Work out the finished part from the listing and answer in its coordinate system (mm). A direction names the side the tool comes from. Give positions to 0.01 mm unless a question says otherwise; leave off trailing zeros. Write each loop counter-clockwise with the first axis right and the second up, starting at its lowest first coordinate (ties: lowest second). Pieces come first, ordered by that corner, then holes. Notation, with made-up numbers: (75, 33) - (130, 33) arc R22 ccw to (130, 57) - close; hole circle Ø5 at (-6.5, 38.5). An arc over 180 degrees is marked (long way). Write item = value, one per line.
from build123d import *

# Parameters (mm, degrees)
BASE_FLANGE1_DEPTH                           = 19.5
SKETCH13_R                                   = 4
CUT_EXTRUDE6_DEPTH                           = 84.228219974
CUT_EXTRUDE7_DEPTH                           = 84.228219974
CUT_EXTRUDE7_DEPTH_BACK                      = 84.228219974
SKETCH33_R                                   = 8
CUT_EXTRUDE10_DEPTH                          = 10
SKETCH34_R                                   = 1.5
CUT_EXTRUDE11_DEPTH                          = 10
BOSS_EXTRUDE1_DEPTH                          = 3
TAB1_START                                   = -3
TAB1_DEPTH                                   = 3
CSK_FOR_M4_COUNTERSUNK_FLAT_HEAD_SCR_2_COUNT = 2
CSK_FOR_M4_COUNTERSUNK_FLAT_HEAD_SCR_2_PITCH = 39.597979746
CSK_FOR_M4_COUNTERSUNK_FLAT_HEAD_SCR_3_COUNT = 2
CSK_FOR_M4_COUNTERSUNK_FLAT_HEAD_SCR_3_PITCH = 56
CSK_FOR_M4_COUNTERSUNK_FLAT_HEAD_SCR_4_COUNT = 2
CSK_FOR_M4_COUNTERSUNK_FLAT_HEAD_SCR_4_PITCH = 39.597979746


# Read off the part's stored shape, not the designer's step: Tab1
# Sheet-metal steps are written as plain solids
with BuildPart() as part:
    # Sketch1 → Base-Flange1 (new, symmetric)
    with BuildSketch(Plane.XY):
        with BuildLine():
            Line((-28.21, 74.65), (-28.21, 2))
            ThreePointArc((-28.21, 2), (-27.624213562, 0.585786438), (-26.21, 0))
            Line((-26.21, 0), (26.21, 0))
            ThreePointArc((26.21, 0), (27.624213562, 0.585786438), (28.21, 2))
            Line((28.21, 2), (28.21, 74.65))
            Line((28.21, 74.65), (31.21, 74.65))
            Line((31.21, 74.65), (31.21, 2))
            ThreePointArc((31.21, 2), (29.745533906, -1.535533906), (26.21, -3))
            Line((26.21, -3), (-26.21, -3))
            ThreePointArc((-26.21, -3), (-29.745533906, -1.535533906), (-31.21, 2))
            Line((-31.21, 2), (-31.21, 74.65))
            Line((-31.21, 74.65), (-28.21, 74.65))
        make_face()
    extrude(amount=BASE_FLANGE1_DEPTH, both=True)

    # Sketch13 → Cut-Extrude6 (cut, through all)
    with BuildSketch(Plane(origin=(0, 0, 0), x_dir=(0, 0, -1), z_dir=(1, 0, 0))):
        with Locations((0, 32)):
            Circle(SKETCH13_R)
    extrude(amount=CUT_EXTRUDE6_DEPTH, mode=Mode.SUBTRACT)

    # Sketch15 → Cut-Extrude7 (cut, two sides: drawn at the far end of the back side and taken through both)
    with BuildSketch(Plane(origin=(0, 0, 0), x_dir=(0, 0, -1), z_dir=(1, 0, 0)).offset(-CUT_EXTRUDE7_DEPTH_BACK)):
        with BuildLine():
            Line((-19.5, 32), (-26.744382408, 32))
            Line((-26.744382408, 32), (-26.744382408, 87.632847334))
            Line((-26.744382408, 87.632847334), (26.744382408, 87.632847334))
            Line((26.744382408, 87.632847334), (26.744382408, 32))
            Line((26.744382408, 32), (19.5, 32))
            ThreePointArc((19.5, 32), (0, 51.5), (-19.5, 32))
        make_face()
        with BuildLine():
            Line((7.470480628, 19.147299148), (10, 14.795349466))
            ThreePointArc((10, 14.795349466), (10.176160856, 13.182152576), (9.097954318, 11.969342816))
            ThreePointArc((9.097954318, 11.969342816), (0, 10), (-9.097954318, 11.969342816))
            ThreePointArc((-9.097954318, 11.969342816), (-10.176160856, 13.182152576), (-10, 14.795349466))
            Line((-10, 14.795349466), (-7.470480628, 19.147299148))
            ThreePointArc((-7.470480628, 19.147299148), (-6.381394917, 20.037080634), (-4.975835097, 19.989959822))
            ThreePointArc((-4.975835097, 19.989959822), (0, 19), (4.975835097, 19.989959822))
            ThreePointArc((4.975835097, 19.989959822), (6.381394917, 20.037080634), (7.470480628, 19.147299148))
        make_face()
    extrude(amount=CUT_EXTRUDE7_DEPTH + CUT_EXTRUDE7_DEPTH_BACK, mode=Mode.SUBTRACT)

    # Sketch33 → Cut-Extrude10 (cut)
    with BuildSketch(Plane(origin=(-28.21, 0, 0), x_dir=(0, 0, -1), z_dir=(1, 0, 0))):
        with Locations((0, 32)):
            Circle(SKETCH33_R)
    extrude(amount=-CUT_EXTRUDE10_DEPTH, mode=Mode.SUBTRACT)

    # Sketch34 → Cut-Extrude11 (cut)
    with BuildSketch(Plane.ZY.offset(31.21)):
        with Locations((-11.490485194, 43.490485194)):
            Circle(SKETCH34_R)
        with Locations((11.490485194, 43.490485194)):
            Circle(SKETCH34_R)
        with Locations((11.490485194, 20.509514806)):
            Circle(SKETCH34_R)
        with Locations((-11.490485194, 20.509514806)):
            Circle(SKETCH34_R)
    extrude(amount=-CUT_EXTRUDE11_DEPTH, mode=Mode.SUBTRACT)

    # Sketch37 → Boss-Extrude1 (add)
    with BuildSketch(Plane.ZY.offset(31.21)):
        with BuildLine():
            Line((7.470480628, 19.147299148), (10, 14.795349466))
            ThreePointArc((10, 14.795349466), (10.176160856, 13.182152576), (9.097954318, 11.969342816))
            ThreePointArc((9.097954318, 11.969342816), (0, 10), (-9.097954318, 11.969342816))
            ThreePointArc((-9.097954318, 11.969342816), (-10.176160856, 13.182152576), (-10, 14.795349466))
            Line((-10, 14.795349466), (-7.470480628, 19.147299148))
            ThreePointArc((-7.470480628, 19.147299148), (-6.381394917, 20.037080634), (-4.975835097, 19.989959822))
            ThreePointArc((-4.975835097, 19.989959822), (0, 19), (4.975835097, 19.989959822))
            ThreePointArc((4.975835097, 19.989959822), (6.381394917, 20.037080634), (7.470480628, 19.147299148))
        make_face()
    extrude(amount=-BOSS_EXTRUDE1_DEPTH)

    # Tab1 outline → Tab1 (add)
    with BuildSketch(Plane.XZ.offset(3).offset(TAB1_START)):
        with BuildLine():
            Line((26.21, 19.5), (26.21, 23.195600876))
            ThreePointArc((26.21, 23.195600876), (0, 35), (-26.21, 23.195600876))
            Line((-26.21, 23.195600876), (-26.21, 19.5))
            Line((-26.21, 19.5), (26.21, 19.5))
        make_face()
        with BuildLine():
            Line((-26.21, -19.5), (-26.21, -23.195600876))
            ThreePointArc((-26.21, -23.195600876), (0, -35), (26.21, -23.195600876))
            Line((26.21, -23.195600876), (26.21, -19.5))
            Line((26.21, -19.5), (-26.21, -19.5))
        make_face()
    extrude(amount=TAB1_DEPTH)

    # Sketch42 → CSK for M4 Countersunk Flat Head Screw1 (revolve, cut)
    with BuildSketch(Plane(origin=(19.798989873, 0, -19.798989873), x_dir=(0, 0, 1), z_dir=(1, 0, 0))):
        Polygon((0, 0), (0, 3), (2.25, 3), (2.25, 2.45), (4.7, 0), align=None)
    csk_for_m4_countersunk_flat_head_screw1 = revolve(axis=Axis((19.798989873, 6.35, -19.798989873), (0, -1, 0)), mode=Mode.SUBTRACT)

    # CSK for M4 Countersunk Flat Head Scr 2: CSK for M4 Countersunk Flat Head Screw1 ×2
    with Locations(*[(-i * CSK_FOR_M4_COUNTERSUNK_FLAT_HEAD_SCR_2_PITCH, 0, 0) for i in range(1, CSK_FOR_M4_COUNTERSUNK_FLAT_HEAD_SCR_2_COUNT)]):
        add(csk_for_m4_countersunk_flat_head_screw1, mode=Mode.SUBTRACT)

    # CSK for M4 Countersunk Flat Head Scr 3: CSK for M4 Countersunk Flat Head Screw1 ×2
    with Locations(*[Vector(-0.7071067811865476, 0, 0.7071067811865476) * (i * CSK_FOR_M4_COUNTERSUNK_FLAT_HEAD_SCR_3_PITCH) for i in range(1, CSK_FOR_M4_COUNTERSUNK_FLAT_HEAD_SCR_3_COUNT)]):
        add(csk_for_m4_countersunk_flat_head_screw1, mode=Mode.SUBTRACT)

    # CSK for M4 Countersunk Flat Head Scr 4: CSK for M4 Countersunk Flat Head Screw1 ×2
    with Locations(*[(0, 0, i * CSK_FOR_M4_COUNTERSUNK_FLAT_HEAD_SCR_4_PITCH) for i in range(1, CSK_FOR_M4_COUNTERSUNK_FLAT_HEAD_SCR_4_COUNT)]):
        add(csk_for_m4_countersunk_flat_head_screw1, mode=Mode.SUBTRACT)


solid = part.part
1. Find section C-C, the plane y = 47. Give the vertices of the cut face in (x, z), then the cut area to 3 significant figures.
Solution:
outline = (-31.21, -12.46) - (-28.21, -12.46) - (-28.21, 12.46) - (-31.21, 12.46) - close; (28.21, -12.46) - (31.21, -12.46) - (31.21, 12.46) - (28.21, 12.46) - close
area = 150 mm^2
2. Find section B-B, the plane y = 33.5. Give the vertices of the cut face in (x, z).
Solution:
outline = (-31.21, -19.44) - (-28.21, -19.44) - (-28.21, -7.86) - (-31.21, -7.86) - close; (-31.21, 7.86) - (-28.21, 7.86) - (-28.21, 19.44) - (-31.21, 19.44) - close; (28.21, -19.44) - (31.21, -19.44) - (31.21, -3.71) - (28.21, -3.71) - close; (28.21, 3.71) - (31.21, 3.71) - (31.21, 19.44) - (28.21, 19.44) - close
3. A tool of negligible diameter and unlimited length cuts with its end or side. For faces 1 (the flat face through (-26.21, -1, 21)), 2 (the cylindrical face through (30, 19, 0)), 3 (the cylindrical face through (-29.731, 19.179, 12.183)), from which of +Z, -Z, +X, -X, +Y, -Y can it reach the whole face along a straight path? Write none if from no direction.
Solution:
face_1 = +Z, -X, +Y, -Y
face_2 = +X
face_3 = -X
4. Given pin 1 (7 mm diameter, centred on x = -19.8, z = 19.8, fed in from +Y); pin 2 (5 mm diameter, centred on x = 19.8, z = -19.8, fed in from +Y); pin 3 (1.5 mm diameter, centred on x = -28, y = 18.5, fed in from -Z), each flat-ended and moving along its own axis, determine where each tip first touches the part or whether it passes through.
Solution:
pin_1 = -1.2
pin_2 = -2.2
pin_3 = -19.5
5. For a pull along Y with two mould halves and no side action, classify faces 4 (the flat face through (26.21, -1, 21)), 5 (the cylindrical face through (-29.731, 42.026, -11.816)), 6 (the cylindrical face through (29.69, 13.2, -10.18)), 7 (the cylindrical face through (-29.731, 51.495, -0.429)) as pulls with the +Y half, pulls with the -Y half, needs draft (parallel to the pull), parting line crosses it, or undercut.
Solution:
face_4 = needs draft
face_5 = undercut
face_6 = undercut
face_7 = pulls with the +Y half
6. Find section D-D, the plane x = 13. Give the vertices of the cut face in (y, z).
Solution:
outline = (-3, -32.5) - (0, -32.5) - (0, 32.5) - (-3, 32.5) - close
7. Find section A-A, the plane z = 0. Give the vertices of the cut face in (x, y), then the cut area to 3 significant figures.
Solution:
outline = (-31.21, 2) arc R5 ccw to (-26.21, -3) - (26.21, -3) arc R5 ccw to (31.21, 2) - (31.21, 10) - (28.21, 10) - (28.21, 2) arc R2 cw to (26.21, 0) - (-26.21, 0) arc R2 cw to (-28.21, 2) - (-28.21, 24) - (-31.21, 24) - close; (-31.21, 40) - (-28.21, 40) - (-28.21, 51.5) - (-31.21, 51.5) - close; (28.21, 19) - (31.21, 19) - (31.21, 28) - (28.21, 28) - close; (28.21, 36) - (31.21, 36) - (31.21, 51.5) - (28.21, 51.5) - close
area = 388 mm^2
8. Straight lines are drawn through the part: line 1 (X direction, y = 31, z = 19); line 2 (Y direction, x = 30, z = 0); line 3 (Z direction, x = 29.95, y = 32). For each, find the intervals that lie inside material, in ascending order.
Solution:
line_1 = -31.21 to -28.21, 28.21 to 31.21
line_2 = -1.26 to 10, 19 to 28, 36 to 51.5
line_3 = -19.5 to -4, 4 to 19.5
